Read the model definition and answer for the solid it produces. Units are mm, in the model's axes. Coordinates: 2 decimals unless noted, no trailing zeros. Loops run counter-clockwise (first coordinate to the right, second up) from the corner with the lowest first, then second, coordinate; pieces in that order, holes last.
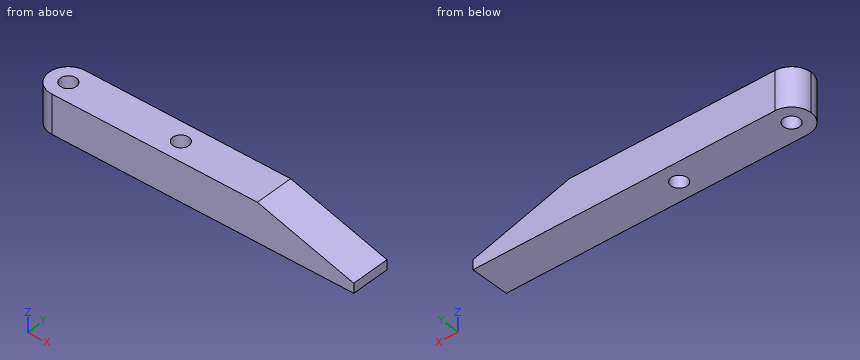
from build123d import *

# Parameters (mm, degrees)
F0_W     = 100
F0_H     = 12
F1_DEPTH = 12
F2_SIZE2 = 9
F2_SIZE  = 30
F3_R     = 5.99999
F5_D     = 5


# Not quite as in the source:
# - a fillet or chamfer is up to 0.001 mm smaller than in the source, because OpenCascade refuses the exact size


with BuildPart() as f1:
    # F0 (on Top) → F1 (new body)
    with BuildSketch(Plane.XY):
        with Locations((50, 6)):
            Rectangle(F0_W, F0_H)
    extrude(amount=F1_DEPTH)

    # F2
    f2_edges = [f1.edges().sort_by_distance(p)[0] for p in [
        (100, 6, 12),
    ]]
    f2_side = f1.faces().sort_by_distance((50, 6, 12))[0]
    chamfer(f2_edges, length=F2_SIZE, length2=F2_SIZE2, reference=f2_side)

    # F3 (radius 6 in the source; OpenCascade refuses exactly that, so slightly less here)
    f3_edges = [f1.edges().sort_by_distance(p)[0] for p in [
        (0, 0, 6),
        (0, 12, 6),
    ]]
    fillet(f3_edges, radius=F3_R)

    # F5 (through all)
    with Locations(Plane.XY.offset(12)):
        with Locations((6, 6), (41, 6)):
            Hole(F5_D / 2)


solid = f1.part
Item 1: A cutting plane is placed at B-B on z = 7.5. Give the number of separate pieces and of enclosed holes in the cut face, then the cut area to 3 significant figures.
Numbers:
separate pieces: 1
enclosed holes: 2
area: 965 mm2
Item 2: A cutting plane is placed at A-A on x = 41. Determine the outline of the cut face in (y, z), then the cut area to 3 significant figures.
Numbers:
outline: (0, 0) - (3.5, 0) - (3.5, 12) - (0, 12) - close; (8.5, 0) - (12, 0) - (12, 12) - (8.5, 12) - close
area: 84.0 mm2
Item 3: Find the intervals of material crossed by line 1 along X through (y, z) = (8, 1.5); line 2 along Y through (x, z) = (41, 6.5); line 3 along X through (y, z) = (6.5, 1.25), in increasing order.
Numbers:
line 1: x = 0.34 to 4.5, 7.5 to 39.5, 42.5 to 100
line 2: y = 0 to 3.5, 8.5 to 12
line 3: x = 0.02 to 3.55, 8.45 to 38.55, 43.45 to 100
Item 4: Given pin 1 (5 mm diameter, centred on y = 10, z = 9.5, fed in from -X); pin 2 (1.5 mm diameter, centred on y = 10.5, z = 6.5, fed in from -X), each flat-ended and moving along its own axis, determine where each tip first touches the part or whether it passes through.
Numbers:
pin 1: stops at x = 0.19
pin 2: stops at x = 1.32
Item 5: A cutting plane is placed at C-C on y = 4.5. Determine the outline of the cut face in (x, z), then the cut area to 3 significant figures.
Numbers:
outline: (0.19, 0) - (4, 0) - (4, 12) - (0.19, 12) - close; (8, 0) - (39, 0) - (39, 12) - (8, 12) - close; (43, 0) - (100, 0) - (100, 3) - (70, 12) - (43, 12) - close
area: 967 mm2
Item 6: A cutting plane is placed at D-D on y = 10. Determine the outline of the cut face in (x, z).
Numbers:
outline: (1.53, 0) - (100, 0) - (100, 3) - (70, 12) - (1.53, 12) - close
